```python
from build123d import *


with BuildPart() as f1:
    # F0 (on Top) → F1 (revolve)
    with BuildSketch(Plane.XY):
        Polygon((12.5, -165), (4, -165), (4, -180), (15, -180), (15, -175), (16, -175), (16, -174), (27, -174), (27, -175), (35, -175), (35, -170), align=None)
        Polygon((4, -160), (4, -165), (12.5, -165), (12.5, 165), (0, 165), (0, -157.690599), align=None)
    revolve(axis=Axis((0, 0, 0), (0, 1, 0)))


solid = f1.part
```
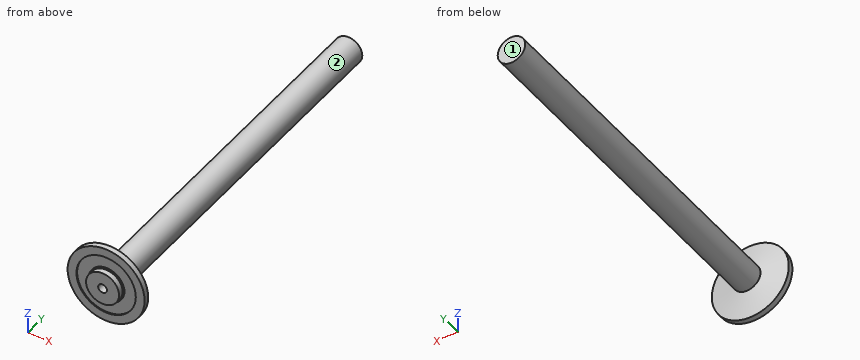
Could you check a few things on this model? Use its own coordinates, in mm. Face numbers are marked on the shaded views. A direction names the side the tool comes from. Round coordinates to 2 decimals unless told otherwise and drop trailing zeros. Write each loop counter-clockwise with the first axis right and the second up, starting at its lowest first coordinate (ties: lowest second). Pieces come first, ordered by that corner, then holes. Notation, with made-up numbers: M 68,35.25 L 82,35.25 A16 ccw 82,49.25 Z; hole C 49.5,28 d9. An arc over 180 degrees is marked long. Answer in a Markdown table with one row per item. Add a question column.
Q1. If I drill on line 1 (X direction, y = -174.7, z = 0); line 2 (X direction, y = -170.25, z = 0), over which ranges is the centre line in solid material (lowest first)? Write a range as from..to.
Q2. Will these pins go through, and if not, where does the flat tip stop? pin 1 Ø1.5 at (y, z) = (107, -11.5) entering from +X; pin 2 Ø8 at (x, z) = (-14, 26.5) entering from -Y; pin 3 Ø5 at (y, z) = (103.5, 8) entering from +X (3 decimals); pin 4 Ø5 at (x, z) = (13, 4) entering from +Y.
Q3. On a 3-axis mill with a long thin cutter (end or side, diameter ignored), from which of +Z, -Z, +X, -X, +Y, -Y can I reach the whole of each face in a straight line? I mean the marked faces 1 and 2. Say none if no direction works.
Q4. Imagine slicing it at A-A (y = -77.5). Please give me the cut outline in (x, z).
Values:
| question | item | result |
|---|---|---|
| 1 | line 1 | -35..-27, -16..-4, 4..16, 27..35 |
| 1 | line 2 | -35..-4, 4..35 |
| 2 | pin 1 | x = 6.38 |
| 2 | pin 2 | y = -175 |
| 2 | pin 3 | x = 11.225 |
| 2 | pin 4 | y = 165 |
| 3 | face 1 | +Z, -Z, +X, -X, +Y |
| 3 | face 2 | +Y |
| 4 | outline | C 0,0 d25 |
